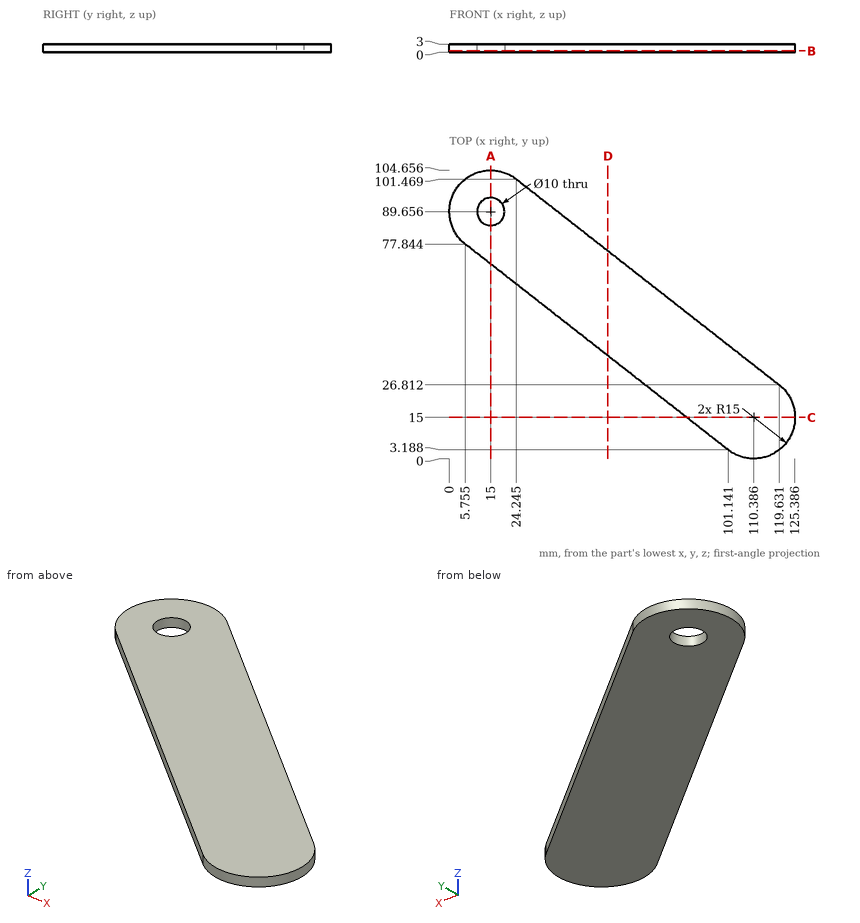
Study the drawing (mm; zero at the part's minimum x, y, z) and answer. Round coordinates to 2 decimals unless told otherwise and drop trailing zeros. Loops run counter-clockwise (first coordinate to the right, second up) from the corner with the lowest first, then second, coordinate; pieces in that order, holes last. Notation, with made-up numbers: M -2,61.25 L 50,61.25 A31 ccw 50,89.25 Z; hole C 13,-32 d9. An arc over 180 degrees is marked long. One line per question, with ' | ' between items.
Q1. Find section A-A, the plane x = 15. Give the vertices of the cut face in (y, z).
Conclusion:
outline: M 70.61,0 L 84.66,0 L 84.66,3 L 70.61,3 Z; M 94.66,0 L 104.66,0 L 104.66,3 L 94.66,3 Z
Q2. Find section C-C, the plane y = 15. Give the vertices of the cut face in (x, z), then the cut area to 3 significant figures.
Conclusion:
outline: M 86.05,0 L 125.39,0 L 125.39,3 L 86.05,3 Z | area: 118 mm2
Q3. This flat-tipped pin is pushed along its axis until it touches: pin 1 Ø1.5 at (x, z) = (45, 0.5) entering from -Y. Where does it stop, or does it pass through?
Conclusion:
pin 1: stops at y = 46.54
Q4. Consider line 1 along Y through (x, z) = (15, 0.75) (1 decimal); line 2 along Y through (x, z) = (17, 1) (1 decimal); line 3 along X through (y, z) = (80, 1.1) (1 decimal). Determine where each line is inside the solid, lowest interval first. Write a range as from..to.
Conclusion:
line 1: y = 70.6..84.7, 94.7..104.7 | line 2: y = 69..85.1, 94.2..104.5 | line 3: x = 3.5..51.7
Q5. Find section B-B, the plane z = 0.5. Give the vertices of the cut face in (x, y) (1 decimal).
Conclusion:
outline: M 5.8,77.8 L 101.1,3.2 A15 ccw 119.6,26.8 L 24.2,101.5 A15 ccw Z; hole C 15,89.7 d10
Q6. Find section D-D, the plane x = 57.5. Give the vertices of the cut face in (y, z) (1 decimal).
Conclusion:
outline: M 37.3,0 L 75.4,0 L 75.4,3 L 37.3,3 Z
